```python
from build123d import *

# Parameters (mm, degrees)
SKETCH1_W           = 1010
SKETCH1_H           = 22.5
BOSS_EXTRUDE1_DEPTH = 2.5
SKETCH2_W           = 1010
SKETCH2_H           = 2.5
BOSS_EXTRUDE2_DEPTH = 25
CUT_EXTRUDE1_DEPTH  = 506.873316652
FILLET1_R           = 1


with BuildPart() as part:
    # Sketch1 → Boss-Extrude1 (new body)
    with BuildSketch(Plane(origin=(0, 0, 0), x_dir=(1, 0, 0), z_dir=(0, 1, 0))):
        Rectangle(SKETCH1_W, SKETCH1_H)
    extrude(amount=BOSS_EXTRUDE1_DEPTH)

    # Sketch2 → Boss-Extrude2 (add)
    with BuildSketch(Plane(origin=(0, 2.5, 0), x_dir=(1, 0, 0), z_dir=(0, 1, 0))):
        with Locations((0, 10)):
            Rectangle(SKETCH2_W, SKETCH2_H)
    extrude(amount=BOSS_EXTRUDE2_DEPTH)

    # Sketch3 → Cut-Extrude1 (cut, through all)
    with BuildSketch(Plane(origin=(0, 0, 0), x_dir=(-1, 0, 0), z_dir=(0, -1, 0))):
        Polygon((505, 11.25), (505, -11.25), (482.5, -11.25), align=None)
        Polygon((-505, 11.25), (-505, -11.25), (-482.5, -11.25), align=None)
    extrude(amount=-CUT_EXTRUDE1_DEPTH, mode=Mode.SUBTRACT)

    # Fillet1
    fillet1_edges = [part.edges().sort_by_distance(p)[0] for p in [
        (0, 27.5, -11.25),
        (0, 27.5, -8.75),
        (0, 2.5, -8.75),
        (0, 0, 11.25),
        (0, 2.5, 11.25),
        (0, 0, -11.25),
    ]]
    fillet(fillet1_edges, radius=FILLET1_R)


solid = part.part
```
The listing builds one solid part. Answer for the finished solid, in the listing's coordinates (mm). A direction names the side the tool comes from. Give positions to 0.01 mm unless a question says otherwise; leave off trailing zeros. Write each loop counter-clockwise with the first axis right and the second up, starting at its lowest first coordinate (ties: lowest second). Pieces come first, ordered by that corner, then holes. Notation, with made-up numbers: (34.25, 74) - (42.25, 74) arc R13 ccw to (42.25, 83) - close; hole circle Ø11 at (75.5, -29). An arc over 180 degrees is marked (long way). Use one line per item in the form item = value. Start each with the question number.
1) Consider line 1 along Z through (x, y) = (339, 12.25); line 2 along X through (y, z) = (5.5, -10.25); line 3 along Y through (x, z) = (-393.5, -3.5). Determine where each line is inside the solid, lowest interval first. Write a range as from..to.
2) A tool of negligible diameter and unlimited length cuts with its end or side. For faces 1 (the face through (-7, 15, -8.75)), 2 (the face through (-7, 14, -11.25)), from which of +Z, -Z, +X, -X, +Y, -Y can it reach the whole face along a straight path? Write none if from no direction.
3) Find section C-C on y = 13.25. Determine the outline of the cut face in (x, z).
4) Find section B-B on z = 5.25. Determine the outline of the cut face in (x, y).
5) Find section A-A on x = -116. Determine the outline of the cut face in (y, z).
6) Flat-ended cylindrical pins translate along their axes: pin 1 Ø10 at (y, z) = (9.5, -5.5) entering from +X; pin 2 Ø1 at (x, y) = (4.5, 24) entering from +Z; pin 3 Ø6 at (y, z) = (12, -6) entering from -X. Find the tip coordinate at first contact, or state that the pin passes through.
Geometry results:
q1.line_1 = -11.25..-8.75
q1.line_2 = -504..504
q1.line_3 = 0..2.5
q2.face_1 = +Z, +X, -X, +Y
q2.face_2 = -Z, +X, -X, +Y, -Y
q3.outline = (-505, -11.25) - (505, -11.25) - (502.5, -8.75) - (-502.5, -8.75) - close
q4.outline = (-488.5, 0) - (488.5, 0) - (488.5, 2.5) - (-488.5, 2.5) - close
q5.outline = (0, -10.25) arc R1 ccw to (1, -11.25) - (26.5, -11.25) arc R1 ccw to (27.5, -10.25) - (27.5, -9.75) arc R1 ccw to (26.5, -8.75) - (3.5, -8.75) arc R1 cw to (2.5, -7.75) - (2.5, 10.25) arc R1 ccw to (1.5, 11.25) - (1, 11.25) arc R1 ccw to (0, 10.25) - close
q6.pin_1 = 504.25
q6.pin_2 = -8.75
q6.pin_3 = -502.75
